The listing builds one solid part. Answer for the finished solid, in the listing's coordinates (mm). A direction names the side the tool comes from. Round coordinates to 2 decimals unless told otherwise and drop trailing zeros. Loops run counter-clockwise (first coordinate to the right, second up) from the corner with the lowest first, then second, coordinate; pieces in that order, holes last. Notation, with made-up numbers: (-6.75, 10) - (34.25, 10) arc R24 ccw to (34.25, 26) - close; hole circle Ø6 at (50.25, 1). An arc over 180 degrees is marked (long way). Write item = value, one per line. Start each with the question number.
1) Section D-D, the plane z = 3.25 is taken. Determine the outline of the cut face in (x, y).
2) Section C-C, the plane z = 15 is taken. Determine the outline of the cut face in (x, y).
3) A tool of negligible diameter and unlimited length cuts with its end or side. For faces 1 (the flat face through (3.4, 12.3, 4)), 2 (the cylindrical face through (-11.923, 3.755, 13.12)), from which of +Z, -Z, +X, -X, +Y, -Y can it reach the whole face along a straight path? Write none if from no direction.
4) Given pin 1 Ø6 at (x, z) = (7, 3) entering from -Y; pin 2 Ø3 at (y, z) = (9.5, 10) entering from +X; pin 3 Ø2 at (x, z) = (-6, 7) entering from -Y, each flat-ended and moving along its own axis, determine where each tip first touches the part or whether it passes through.
5) Straight lines are drawn through the part: line 1 along Y through (x, z) = (0, 9.5); line 2 along Y through (x, z) = (0, 1.3); line 3 along Z through (x, y) = (-3, 13.5). For each, find the intervals that lie inside material, in ascending order.
6) Section A-A, the plane y = 0 is taken. Determine the outline of the cut face in (x, z), and give its area (4 significant figures).
7) For a pull along X with two mould halves and no side action, classify faces 3 (the cylindrical face through (-3.47, -15.62, 11.09)), 4 (the flat face through (-10, -8, 22.5)), 5 (the cylindrical face through (14.985, 0.66, 1.972)) as released by +X, released by -X, zero draft, split by the parting line, or undercut.
from build123d import *

# Parameters (mm, degrees)
SKETCH_1_R          = 16
EXTRUDE_1_DEPTH     = 22.5
SKETCH_2_R          = 15
CUT_EXTRUDE_3_DEPTH = 4
SKETCH_3_R          = 12.5
CUT_EXTRUDE_4_DEPTH = 19.5


with BuildPart() as part:
    # Эскиз1 → Вытянуть1 (new body)
    with BuildSketch(Plane.XY):
        Circle(SKETCH_1_R)
    extrude(amount=EXTRUDE_1_DEPTH)

    # Эскиз2 → Вытянуть3 (cut)
    with BuildSketch(Plane(origin=(0, 0, 0), x_dir=(-1, 0, 0), z_dir=(0, 0, -1))):
        Circle(SKETCH_2_R)
    extrude(amount=-CUT_EXTRUDE_3_DEPTH, mode=Mode.SUBTRACT)

    # Эскиз3 → Вытянуть4 (cut, through all)
    with BuildSketch(Plane(origin=(0, 0, 4), x_dir=(-1, 0, 0), z_dir=(0, 0, -1))):
        Circle(SKETCH_3_R)
    extrude(amount=-CUT_EXTRUDE_4_DEPTH, mode=Mode.SUBTRACT)


solid = part.part
Geometry check:
q1.outline = circle Ø32 at (0, 0); hole circle Ø30 at (0, 0)
q2.outline = circle Ø32 at (0, 0); hole circle Ø25 at (0, 0)
q3.face_1 = -Z
q3.face_2 = +Z, -Z
q4.pin_1 = -15.49
q4.pin_2 = 13.86
q4.pin_3 = -15.2
q5.line_1 = -16 to -12.5, 12.5 to 16
q5.line_2 = -16 to -15, 15 to 16
q5.line_3 = 4 to 22.5
q6.outline = (-16, 0) - (-15, 0) - (-15, 4) - (-12.5, 4) - (-12.5, 22.5) - (-16, 22.5) - close; (12.5, 4) - (15, 4) - (15, 0) - (16, 0) - (16, 22.5) - (12.5, 22.5) - close
q6.area = 137.5 mm2
q7.face_3 = split by the parting line
q7.face_4 = zero draft
q7.face_5 = undercut
